Could you check a few things on this model? Use its own coordinates, in mm. Face numbers are marked on the shaded views. Coordinates: 2 decimals unless noted, no trailing zeros. Order: outer loops, then holes, each group sorted by start corner. A loop starts at its lowest first (then second) coordinate and runs counter-clockwise, first axis right, second up. Notation, with made-up numbers: M -0.75,47.5 L 39.25,47.5 A22 ccw 39.25,69.5 Z; hole C 26,-28 d9. An arc over 180 degrees is marked long. One line per question, with ' | ' between items. Start each with the question number.
from build123d import *

# Parameters (mm, degrees)
BOSS_EXTRUDE1_START = 5.5
SKETCH4_W           = 13.614691885
SKETCH4_H           = 1.5
BOSS_EXTRUDE1_DEPTH = 15


with BuildPart() as part:
    # Sketch1 → Revolve1 (revolve)
    with BuildSketch(Plane.XY):
        with BuildLine():
            Line((-20, 26), (-27.5, 26))
            Line((-27.5, 26), (-27.5, 25))
            Line((-27.5, 25), (-24.9, 25))
            ThreePointArc((-24.9, 25), (-23.057568057, 13), (-24.9, 1))
            Line((-24.9, 1), (-27.5, 1))
            Line((-27.5, 1), (-27.5, 0))
            Line((-27.5, 0), (-20, 0))
            Line((-20, 0), (-20, 5.5))
            Line((-20, 5.5), (-20, 20.5))
            Line((-20, 20.5), (-20, 26))
        make_face()
        Polygon((-4.5, 26), (-4.5, 0), (-7.5, 0), (-7.5, 5.5), (-7.5, 20.5), (-7.5, 26.037065381), align=None)
    revolve(axis=Axis((0, 42.404735677, 0), (0, -1, 0)))

    # Sketch4 → Boss-Extrude1 (add)
    with BuildSketch(Plane(origin=(0, 0, 0), x_dir=(1, 0, 0), z_dir=(0, 1, 0)).offset(BOSS_EXTRUDE1_START)):
        with Locations((13.641384633, 0)):
            Rectangle(SKETCH4_W, SKETCH4_H)
        Polygon((4.066538398, -5.543451116), (10.873884341, -17.334120153), (9.574846235, -18.084120153), (2.767500292, -6.293451116), align=None)
        Polygon((-2.767500292, -6.293451116), (-9.574846235, -18.084120153), (-10.873884341, -17.334120153), (-4.066538398, -5.543451116), align=None)
        with Locations((-13.641384633, 0)):
            Rectangle(SKETCH4_W, SKETCH4_H)
        Polygon((-4.066538398, 5.543451116), (-10.873884341, 17.334120153), (-9.574846235, 18.084120153), (-2.767500292, 6.293451116), align=None)
        Polygon((2.767500292, 6.293451116), (9.574846235, 18.084120153), (10.873884341, 17.334120153), (4.066538398, 5.543451116), align=None)
    extrude(amount=BOSS_EXTRUDE1_DEPTH)


solid = part.part
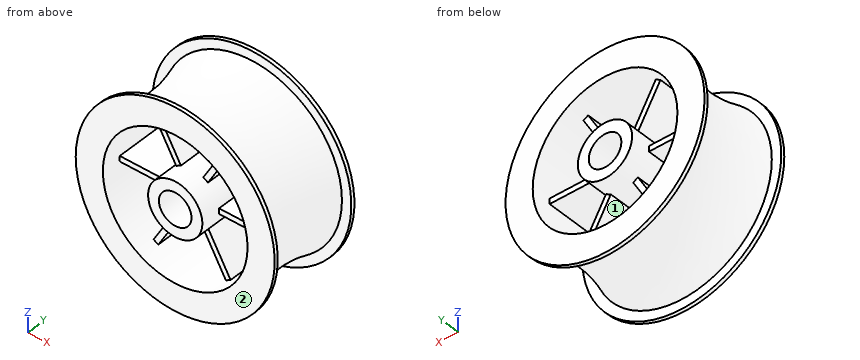
(1) If I drill on line 1 along Y through (x, z) = (-8, 25); line 2 along X through (y, z) = (8.5, 14); line 3 along Z through (x, y) = (0, 15.75), over which ranges is the centre line in solid material (lowest first)? Write a range as from..to.
(2) Imagine slicing it at B-B, the plane x = 0. Write out the boundary of the cut face in (y, z).
(3) Imagine slicing it at C-C, the plane y = 8.75. Write out the boundary of the cut face in (x, z), plus the area to 3 significant figures.
(4) Imagine slicing it at D-D, the plane y = 4.5. Write out the boundary of the cut face in (x, z), plus the area to 3 significant figures.
(5) For P1, Ø4, axis at x = -7.5, z = -13, coming from the +Y side; P2, Ø3, axis at y = 18, z = 8.5, coming from the -X side; P3, Ø5, axis at y = 14, z = 1.5, coming from the +X side, each with a flat end and sliding along its axis, tell me the tip position at first contact or that it passes through.
(6) We'd pull the mould along X, two halves only. Please class the marked faces 1 and 2: +X half, -X half, draft (parallel to the pull), parting line (faces both ways), or undercut.
Answers:
1) line 1: 0..1, 25..26 | line 2: -18.64..-14.28, -8.95..-7.22, 7.22..8.95, 14.28..18.64 | line 3: -23.15..-20, -7.5..-4.5, 4.5..7.5, 20..23.15
2) outline: M 0,-27.5 L 1,-27.5 L 1,-24.9 A40 cw 25,-24.9 L 25,-27.5 L 26,-27.5 L 26,-20 L 0,-20 Z; M 0,-7.5 L 26.04,-7.5 L 26,-4.5 L 0,-4.5 Z; M 0,4.5 L 26,4.5 L 26.04,7.5 L 0,7.5 Z; M 0,20 L 26,20 L 26,27.5 L 25,27.5 L 25,24.9 A40 cw 1,24.9 L 1,27.5 L 0,27.5 Z
3) outline: C 0,0 d46.57; hole M -19.99,-0.75 A20 ccw -10.64,-16.93 L -4.38,-6.09 A7.5 cw -7.46,-0.75 Z; hole M -19.99,0.75 L -7.46,0.75 A7.5 cw -4.38,6.09 L -10.64,16.93 A20 ccw Z; hole M -9.34,-17.68 A20 ccw 9.34,-17.68 L 3.08,-6.84 A7.5 cw -3.08,-6.84 Z; hole M -9.34,17.68 L -3.08,6.84 A7.5 cw 3.08,6.84 L 9.34,17.68 A20 ccw Z; hole C 0,0 d9; hole M 4.38,-6.09 L 10.64,-16.93 A20 ccw 19.99,-0.75 L 7.46,-0.75 A7.5 cw Z; hole M 4.38,6.09 A7.5 cw 7.46,0.75 L 19.99,0.75 A20 ccw 10.64,16.93 Z | area: 672 mm²
4) outline: C 0,0 d47.94; C 0,0 d15; hole C 0,0 d40; hole C 0,0 d9 | area: 662 mm²
5) P1: y = 20.5 | P2: x = -22.34 | P3: x = 23.19
6) face 1: undercut | face 2: draft
